For this review, take the finished solid that the model builds, in its own axes (mm). Face numbers are marked on the shaded views. Coordinates: 2 decimals unless noted, no trailing zeros. Order: outer loops, then holes, each group sorted by start corner. A loop starts at its lowest first (then second) coordinate and runs counter-clockwise, first axis right, second up. Notation, with made-up numbers: (50, 53.5) -> (69, 53.5) arc R14 cw to (69, 58.5) -> close; hole circle Ø7 at (69.25, -13). An arc over 180 degrees is marked (long way). Return JSON: item names as keys, results as strings. Group by question number.
Item 1: Draft analysis for pull direction X (two halves, no side actions). For the marked faces 1, 2 and 3, state which applies: +X half, -X half, draft (parallel to the pull), parting line (faces both ways), or undercut.
Item 2: Insertion check: pin 1 (10 mm diameter, centred on y = -499, z = 432, fed in from -X); pin 2 (0.8 mm diameter, centred on x = -162, z = 433.5, fed in from +Y); pin 3 (2 mm diameter, centred on y = -510.5, z = 434, fed in from +X). Each pin has a flat end and moves straight along its axis. Give the tip position at first contact, or say it passes through.
Item 3: Take a section at D-D (z = 445). Write out the cut boundary in (x, y).
Item 4: For line 1 along X through (y, z) = (-511.5, 441); line 2 along Y through (x, z) = (-135, 432); line 3 along Y through (x, z) = (-116.5, 449), list the stretches that pass through material, from the lowest coordinate up.
Item 5: Take a section at C-C (z = 430). Count the separate pieces of the cut face and the enclosed holes in it, then the cut area to 3 significant figures.
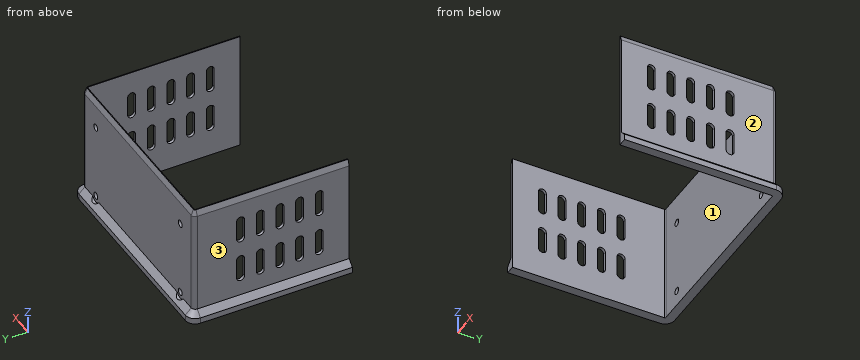
```python
from build123d import *
from OCP.BRepFilletAPI import BRepFilletAPI_MakeChamfer

# Parameters (mm, degrees)
BOSS_EXTRUDE1_DEPTH = 61.5
CHAMFER1_SIZE       = 3
CHAMFER1_SIZE2      = 1.091910703
SKETCH4_R           = 1.75
CUT_EXTRUDE1_DEPTH  = 10
BOSS_EXTRUDE2_DEPTH = 3
CHAMFER2_SIZE       = 3
CUT_EXTRUDE2_DEPTH  = 145
SKETCH7_R           = 3.5
CUT_EXTRUDE3_DEPTH  = 10


with BuildPart() as part:
    # Sketch3 → Boss-Extrude1 (new body)
    with BuildSketch(Plane.XY.offset(389.620141885)):
        with BuildLine():
            Line((-161.210843614, -470.098939869), (-61.210843614, -470.098939869))
            ThreePointArc((-61.210843614, -470.098939869), (-60.857290223, -470.245386479), (-60.710843614, -470.598939869))
            Line((-60.710843614, -470.598939869), (-60.710843614, -547.798939869))
            Line((-60.710843614, -547.798939869), (-59.210843614, -547.798939869))
            Line((-59.210843614, -547.798939869), (-59.210843614, -470.598939869))
            ThreePointArc((-59.210843614, -470.598939869), (-59.796630051, -469.184726307), (-61.210843614, -468.598939869))
            Line((-61.210843614, -468.598939869), (-161.210843614, -468.598939869))
            ThreePointArc((-161.210843614, -468.598939869), (-162.625057176, -469.184726307), (-163.210843614, -470.598939869))
            Line((-163.210843614, -470.598939869), (-163.210843614, -547.798939869))
            Line((-163.210843614, -547.798939869), (-161.710843614, -547.798939869))
            Line((-161.710843614, -547.798939869), (-161.710843614, -544.99774542))
            Line((-161.710843614, -544.99774542), (-161.710843614, -470.598939869))
            ThreePointArc((-161.710843614, -470.598939869), (-161.564397004, -470.245386479), (-161.210843614, -470.098939869))
        make_face()
    extrude(amount=BOSS_EXTRUDE1_DEPTH)

    # Chamfer1: one chamfer whose edges measure the first distance from different faces: ONE call of the kernel's chamfer builder (chamfer() names one face for all edges)
    chamfer1_edges_1 = [part.edges().sort_by_distance(p)[0] for p in [
        (-59.796630051, -469.184726307, 451.120141885),
    ]]
    chamfer1_side_1 = [part.faces().sort_by_distance(p)[0] for p in [
        (-59.796630051, -469.184726307, 420.370141885),
    ]]
    chamfer1_edges_2 = [part.edges().sort_by_distance(p)[0] for p in [
        (-111.210843614, -468.598939869, 451.120141885),
    ]]
    chamfer1_side_2 = [part.faces().sort_by_distance(p)[0] for p in [
        (-111.210843614, -468.598939869, 420.370141885),
    ]]
    chamfer1_edges_3 = [part.edges().sort_by_distance(p)[0] for p in [
        (-162.625057176, -469.184726307, 451.120141885),
    ]]
    chamfer1_side_3 = [part.faces().sort_by_distance(p)[0] for p in [
        (-162.625057176, -469.184726307, 420.370141885),
    ]]
    chamfer1_edges_4 = [part.edges().sort_by_distance(p)[0] for p in [
        (-163.210843614, -509.198939869, 451.120141885),
    ]]
    chamfer1_side_4 = [part.faces().sort_by_distance(p)[0] for p in [
        (-163.210843614, -509.198939869, 420.370141885),
    ]]
    chamfer1_edges_5 = [part.edges().sort_by_distance(p)[0] for p in [
        (-59.210843614, -509.198939869, 451.120141885),
    ]]
    chamfer1_side_5 = [part.faces().sort_by_distance(p)[0] for p in [
        (-59.210843614, -509.198939869, 420.370141885),
    ]]
    chamfer1 = BRepFilletAPI_MakeChamfer(part.part.solid().wrapped)
    for e in chamfer1_edges_1:
        chamfer1.Add(CHAMFER1_SIZE, CHAMFER1_SIZE2, e.wrapped, chamfer1_side_1[0].wrapped)  # the first distance lies on this face
    for e in chamfer1_edges_2:
        chamfer1.Add(CHAMFER1_SIZE, CHAMFER1_SIZE2, e.wrapped, chamfer1_side_2[0].wrapped)  # the first distance lies on this face
    for e in chamfer1_edges_3:
        chamfer1.Add(CHAMFER1_SIZE, CHAMFER1_SIZE2, e.wrapped, chamfer1_side_3[0].wrapped)  # the first distance lies on this face
    for e in chamfer1_edges_4:
        chamfer1.Add(CHAMFER1_SIZE, CHAMFER1_SIZE2, e.wrapped, chamfer1_side_4[0].wrapped)  # the first distance lies on this face
    for e in chamfer1_edges_5:
        chamfer1.Add(CHAMFER1_SIZE, CHAMFER1_SIZE2, e.wrapped, chamfer1_side_5[0].wrapped)  # the first distance lies on this face
    add(Compound.cast(chamfer1.Shape()), mode=Mode.REPLACE)

    # Sketch4 → Cut-Extrude1 (cut)
    with BuildSketch(Plane(origin=(0, -468.598939869, 0), x_dir=(1, 0, 0), z_dir=(0, 1, 0))):
        with Locations(Location((-150.910843614, -397.620141885, 0), (0, 0, 270))):
            Circle(SKETCH4_R)
        with Locations(Location((-71.510843614, -397.620141885, 0), (0, 0, 270))):
            Circle(SKETCH4_R)
        with Locations(Location((-71.510843614, -436.241358014, 0), (0, 0, 270))):
            Circle(SKETCH4_R)
        with Locations(Location((-150.910843614, -436.241358014, 0), (0, 0, 270))):
            Circle(SKETCH4_R)
    extrude(amount=-CUT_EXTRUDE1_DEPTH, mode=Mode.SUBTRACT)

    # Sketch5 → Boss-Extrude2 (add)
    with BuildSketch(Plane(origin=(0, 0, 389.620141885), x_dir=(-1, 0, 0), z_dir=(0, 0, -1))):
        with BuildLine():
            Line((59.310843614, -547.798939869), (59.310843614, -470.598939869))
            ThreePointArc((59.310843614, -470.598939869), (59.867340729, -469.255436985), (61.210843614, -468.698939869))
            Line((61.210843614, -468.698939869), (161.210843614, -468.698939869))
            ThreePointArc((161.210843614, -468.698939869), (162.554346498, -469.255436985), (163.110843614, -470.598939869))
            Line((163.110843614, -470.598939869), (163.110843614, -547.798939869))
            Line((163.110843614, -547.798939869), (166.210843614, -547.798939869))
            Line((166.210843614, -547.798939869), (166.210843614, -470.598939869))
            ThreePointArc((166.210843614, -470.598939869), (164.74637752, -467.063405963), (161.210843614, -465.598939869))
            Line((161.210843614, -465.598939869), (61.210843614, -465.598939869))
            ThreePointArc((61.210843614, -465.598939869), (57.675309708, -467.063405963), (56.210843614, -470.598939869))
            Line((56.210843614, -470.598939869), (56.210843614, -547.798939869))
            Line((56.210843614, -547.798939869), (59.310843614, -547.798939869))
        make_face()
    extrude(amount=-BOSS_EXTRUDE2_DEPTH)

    # Chamfer2
    chamfer2_edges = [part.edges().sort_by_distance(p)[0] for p in [
        (-163.210843614, -509.198939869, 392.620141885),
        (-162.625057176, -469.184726307, 392.620141885),
        (-111.210843614, -468.598939869, 392.620141885),
        (-59.796630051, -469.184726307, 392.620141885),
        (-59.210843614, -509.198939869, 392.620141885),
    ]]
    chamfer(chamfer2_edges, length=CHAMFER2_SIZE - 0.0001)  # a hair under: the kernel refuses the full size

    # Sketch6 → Cut-Extrude2 (cut)
    with BuildSketch(Plane(origin=(-59.210843614, 0, 0), x_dir=(0, 0, -1), z_dir=(1, 0, 0))):
        with BuildLine():
            Line((-437.620141885, -490.598939869), (-427.620141885, -490.598939869))
            ThreePointArc((-427.620141885, -490.598939869), (-425.620141885, -492.598939869), (-427.620141885, -494.598939869))
            Line((-427.620141885, -494.598939869), (-437.620141885, -494.598939869))
            ThreePointArc((-437.620141885, -494.598939869), (-439.620141885, -492.598939869), (-437.620141885, -490.598939869))
        make_face()
        with BuildLine():
            Line((-415.620141885, -490.598939869), (-405.620141885, -490.598939869))
            ThreePointArc((-405.620141885, -490.598939869), (-403.620141885, -492.598939869), (-405.620141885, -494.598939869))
            Line((-405.620141885, -494.598939869), (-415.620141885, -494.598939869))
            ThreePointArc((-415.620141885, -494.598939869), (-417.620141885, -492.598939869), (-415.620141885, -490.598939869))
        make_face()
        with BuildLine():
            Line((-437.620141885, -500.598939869), (-427.620141885, -500.598939869))
            ThreePointArc((-427.620141885, -500.598939869), (-425.620141885, -502.598939869), (-427.620141885, -504.598939869))
            Line((-427.620141885, -504.598939869), (-437.620141885, -504.598939869))
            ThreePointArc((-437.620141885, -504.598939869), (-439.620141885, -502.598939869), (-437.620141885, -500.598939869))
        make_face()
        with BuildLine():
            Line((-415.620141885, -500.598939869), (-405.620141885, -500.598939869))
            ThreePointArc((-405.620141885, -500.598939869), (-403.620141885, -502.598939869), (-405.620141885, -504.598939869))
            Line((-405.620141885, -504.598939869), (-415.620141885, -504.598939869))
            ThreePointArc((-415.620141885, -504.598939869), (-417.620141885, -502.598939869), (-415.620141885, -500.598939869))
        make_face()
        with BuildLine():
            Line((-437.620141885, -510.598939869), (-427.620141885, -510.598939869))
            ThreePointArc((-427.620141885, -510.598939869), (-425.620141885, -512.598939869), (-427.620141885, -514.598939869))
            Line((-427.620141885, -514.598939869), (-437.620141885, -514.598939869))
            ThreePointArc((-437.620141885, -514.598939869), (-439.620141885, -512.598939869), (-437.620141885, -510.598939869))
        make_face()
        with BuildLine():
            Line((-415.620141885, -510.598939869), (-405.620141885, -510.598939869))
            ThreePointArc((-405.620141885, -510.598939869), (-403.620141885, -512.598939869), (-405.620141885, -514.598939869))
            Line((-405.620141885, -514.598939869), (-415.620141885, -514.598939869))
            ThreePointArc((-415.620141885, -514.598939869), (-417.620141885, -512.598939869), (-415.620141885, -510.598939869))
        make_face()
        with BuildLine():
            Line((-437.620141885, -520.598939869), (-427.620141885, -520.598939869))
            ThreePointArc((-427.620141885, -520.598939869), (-425.620141885, -522.598939869), (-427.620141885, -524.598939869))
            Line((-427.620141885, -524.598939869), (-437.620141885, -524.598939869))
            ThreePointArc((-437.620141885, -524.598939869), (-439.620141885, -522.598939869), (-437.620141885, -520.598939869))
        make_face()
        with BuildLine():
            Line((-415.620141885, -520.598939869), (-405.620141885, -520.598939869))
            ThreePointArc((-405.620141885, -520.598939869), (-403.620141885, -522.598939869), (-405.620141885, -524.598939869))
            Line((-405.620141885, -524.598939869), (-415.620141885, -524.598939869))
            ThreePointArc((-415.620141885, -524.598939869), (-417.620141885, -522.598939869), (-415.620141885, -520.598939869))
        make_face()
        with BuildLine():
            Line((-437.620141885, -530.598939869), (-427.620141885, -530.598939869))
            ThreePointArc((-427.620141885, -530.598939869), (-425.620141885, -532.598939869), (-427.620141885, -534.598939869))
            Line((-427.620141885, -534.598939869), (-437.620141885, -534.598939869))
            ThreePointArc((-437.620141885, -534.598939869), (-439.620141885, -532.598939869), (-437.620141885, -530.598939869))
        make_face()
        with BuildLine():
            Line((-415.620141885, -530.598939869), (-405.620141885, -530.598939869))
            ThreePointArc((-405.620141885, -530.598939869), (-403.620141885, -532.598939869), (-405.620141885, -534.598939869))
            Line((-405.620141885, -534.598939869), (-415.620141885, -534.598939869))
            ThreePointArc((-415.620141885, -534.598939869), (-417.620141885, -532.598939869), (-415.620141885, -530.598939869))
        make_face()
    extrude(amount=-CUT_EXTRUDE2_DEPTH, mode=Mode.SUBTRACT)

    # Sketch7 → Cut-Extrude3 (cut)
    with BuildSketch(Plane(origin=(0, -468.598939869, 0), x_dir=(1, 0, 0), z_dir=(0, 1, 0))):
        with Locations((-150.910843614, -397.620141885)):
            Circle(SKETCH7_R)
        with Locations((-71.510843614, -397.620141885)):
            Circle(SKETCH7_R)
    extrude(amount=CUT_EXTRUDE3_DEPTH, mode=Mode.SUBTRACT)


solid = part.part
```
Findings below:
{
 "1": {"face 1": "undercut", "face 2": "+X half", "face 3": "-X half"},
 "2": {"pin 1": "stops at x = -163.21", "pin 2": "stops at y = -468.64", "pin 3": "stops at x = -59.21"},
 "3": {"outline": "(-163.21, -547.8) -> (-161.71, -547.8) -> (-161.71, -470.6) arc R0.5 cw to (-161.21, -470.1) -> (-61.21, -470.1) arc R0.5 cw to (-60.71, -470.6) -> (-60.71, -547.8) -> (-59.21, -547.8) -> (-59.21, -470.6) arc R2 ccw to (-61.21, -468.6) -> (-161.21, -468.6) arc R2 ccw to (-163.21, -470.6) -> close"},
 "4": {"line 1": "x = -163.21 to -161.71, -60.71 to -59.21", "line 2": "y = -470.1 to -468.6", "line 3": "y = -470.1 to -468.92"},
 "5": {"separate pieces": "11", "enclosed holes": "0", "area": "327 mm2"}
}
